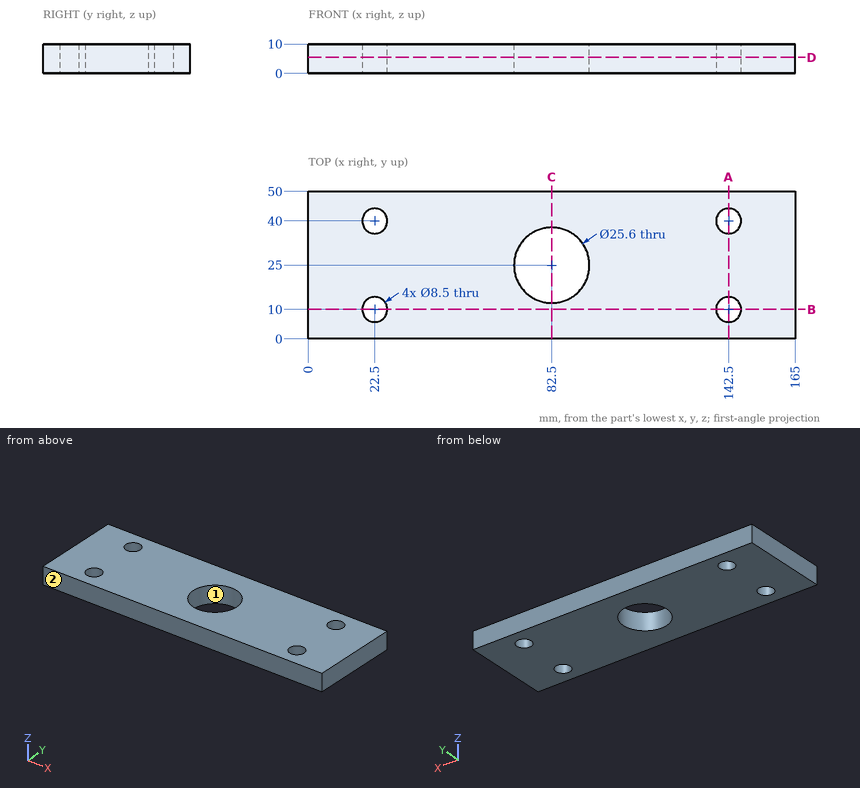
Job drawing, mm, ordinate dimensions from the low corner. One solid piece. Give positions to 0.01 mm unless a question says otherwise; leave off trailing zeros. Loops run counter-clockwise (first coordinate to the right, second up) from the corner with the lowest first, then second, coordinate; pieces in that order, holes last. Notation, with made-up numbers: M 19.5,1 L 24.5,1 A38 ccw 24.5,40 Z; hole C -17.75,86 d7. An arc over 180 degrees is marked long. Put each result on its own line as item: value. Start each with the question number.
1) Probe probe 1 along Y at (x, z) = (142.5, 4.75); probe 2 along X at (y, z) = (7.5, 6.5); probe 3 along X at (y, z) = (36.5, 2). List the from-to ranges inside material, lowest first.
2) Pull direction X, two halves, no side cores. Call the marked faces 1 and 2: +X half, -X half, draft (parallel to the pull), parting line (faces both ways), or undercut.
3) Saw through at C-C (x = 82.5). List the corners of the cut face in (y, z), then the cut area to 3 significant figures.
4) Saw through at A-A (x = 142.5). List the corners of the cut face in (y, z), then the cut area to 3 significant figures.
5) Saw through at D-D (z = 5.5). List the corners of the cut face in (x, y).
6) Saw through at B-B (y = 10). List the corners of the cut face in (x, z).
Numbers:
1. probe 1: 0 to 5.75, 14.25 to 35.75, 44.25 to 50
1. probe 2: 0 to 19.06, 25.94 to 139.06, 145.94 to 165
1. probe 3: 0 to 20.09, 24.91 to 76.88, 88.12 to 140.09, 144.91 to 165
2. face 1: undercut
2. face 2: draft
3. outline: M 0,0 L 12.2,0 L 12.2,10 L 0,10 Z; M 37.8,0 L 50,0 L 50,10 L 37.8,10 Z
3. area: 244 mm^2
4. outline: M 0,0 L 5.75,0 L 5.75,10 L 0,10 Z; M 14.25,0 L 35.75,0 L 35.75,10 L 14.25,10 Z; M 44.25,0 L 50,0 L 50,10 L 44.25,10 Z
4. area: 330 mm^2
5. outline: M 0,0 L 165,0 L 165,50 L 0,50 Z; hole C 22.5,10 d8.5; hole C 22.5,40 d8.5; hole C 82.5,25 d25.6; hole C 142.5,10 d8.5; hole C 142.5,40 d8.5
6. outline: M 0,0 L 18.25,0 L 18.25,10 L 0,10 Z; M 26.75,0 L 138.25,0 L 138.25,10 L 26.75,10 Z; M 146.75,0 L 165,0 L 165,10 L 146.75,10 Z
